Autodesk Inventor part; units mm, degrees
ref_plane "Work Plane1" through (-16.6341, -25.631, 0) normal (0, 0, 1) x (1, 0, 0)
ref_plane "YZ Plane" through (0, 0, 0) normal (1, 0, 0) x (0, 1, 0)
ref_plane "XZ Plane" through (0, 0, 0) normal (0, 1, 0) x (-1, 0, 0)
sketch "Sketch1" plane through (0, 0, 0) normal (0, 1, 0) x (-1, 0, 0)
  line L0 (5.5341, -4.8619) -> (4.7341, -5.0029)
  line L1 (5.5341, -4.4619) -> (5.5341, -4.8619)
  line L2 (4.7341, -4) -> (5.5341, -4.4619)
  line L3 (4.7341, -3.0029) -> (4.7341, -4)
  line L4 (5.5341, -2.8619) -> (4.7341, -3.0029)
  line L5 (5.5341, -2.4619) -> (5.5341, -2.8619)
  line L6 (4.7341, -2) -> (5.5341, -2.4619)
  line L7 (4.7341, -1.0029) -> (4.7341, -2)
  line L8 (5.5341, -0.8619) -> (4.7341, -1.0029)
  line L9 (5.5341, -0.4619) -> (5.5341, -0.8619)
  line L10 (4.7341, 0) -> (5.5341, -0.4619)
  line L11 (10.1341, 0) -> (4.7341, 0)
  line L12 (9.3341, -0.4619) -> (10.1341, 0)
  line L13 (9.3341, -0.8619) -> (9.3341, -0.4619)
  line L14 (10.1341, -1.0029) -> (9.3341, -0.8619)
  line L15 (10.1341, -1.0029) -> (10.1341, -2)
  line L16 (9.3341, -2.4619) -> (10.1341, -2)
  line L17 (9.3341, -2.8619) -> (9.3341, -2.4619)
  line L18 (10.1341, -3.0029) -> (9.3341, -2.8619)
  line L19 (10.1341, -3.0029) -> (10.1341, -4)
  line L20 (9.3341, -4.4619) -> (10.1341, -4)
  line L21 (9.3341, -4.8619) -> (9.3341, -4.4619)
  line L22 (10.1341, -5.0029) -> (9.3341, -4.8619)
  line L23 (10.1341, -5.0029) -> (10.1341, -6)
  line L24 (9.3341, -6.4619) -> (10.1341, -6)
  line L25 (9.3341, -6.8619) -> (9.3341, -6.4619)
  line L26 (10.1341, -7.0029) -> (9.3341, -6.8619)
  line L27 (10.1341, -7.0029) -> (10.1341, -8)
  line L28 (9.3341, -8.4619) -> (10.1341, -8)
  line L29 (9.3341, -8.8619) -> (9.3341, -8.4619)
  line L30 (10.1336, -9.0029) -> (9.3341, -8.8619)
  line L31 (10.1341, -9) -> (10.1341, -10.8672)
  arc A0 (10.1341, -10.8672) -> (10.1663, -11.225) centre (12.1341, -10.8672) ccw
  line L32 (4.5189, -11.225) -> (10.1663, -11.225)
  arc A1 (4.5189, -11.225) -> (4.7341, -10.3226) centre (2.7341, -10.3226) ccw
  line L33 (4.7341, -9) -> (4.7341, -10.3226)
  line L34 (5.5341, -8.8619) -> (4.7346, -9.0029)
  line L35 (5.5341, -8.4619) -> (5.5341, -8.8619)
  line L36 (4.7341, -8) -> (5.5341, -8.4619)
  line L37 (4.7341, -7.0029) -> (4.7341, -8)
  line L38 (5.5341, -6.8619) -> (4.7341, -7.0029)
  line L39 (5.5341, -6.4619) -> (5.5341, -6.8619)
  line L40 (4.7341, -6) -> (5.5341, -6.4619)
  line L41 (4.7341, -5.0029) -> (4.7341, -6)
  line L42 (10.1341, 0) -> (8.6341, 0)
  line L43 (4.7341, 0) -> (6.2341, 0)
  line L44 (6.2341, 0) -> (6.2341, -6)
  line L45 (6.2341, -6) -> (8.6341, -6)
  line L46 (8.6341, -6) -> (8.6341, 0)
  line L47 (8.6341, -6) -> (8.3837, -8.8619)
  line L48 (8.6341, -6) -> (11.5069, -6) construction
  line L49 (6.2341, -6) -> (6.4845, -8.8619)
  line L50 (6.2341, -6) -> (9.1069, -6) construction
  line L51 (6.4845, -8.8619) -> (8.3837, -8.8619)
  line L52 (8.3837, -8.8619) -> (8.2259, -10.666)
  line L53 (8.2259, -10.666) -> (8.1769, -11.225)
  line L54 (6.4845, -8.8619) -> (6.6912, -11.225)
  line L55 (8.6341, 0) -> (6.2341, 0)
  line L56 (6.2341, 0) -> (6.2341, 2)
  line L57 (6.2341, 2) -> (8.6341, 2)
  line L58 (8.6341, 2) -> (8.6341, 0)
  point P0 (0, 0)
  dimension "d0" = 1.5
  dimension "d1" = 1.5
  dimension "d2" = 6
  dimension "d3" = 95
  dimension "d4" = 85
  dimension "d5" = 2
extrude "Extrusion1" add sketch "Sketch1" against normal blind 6.6 contours L56 L57 L58 L11 | L11 L46 L45 L44 | L54 L51 L52 L53 L32 | L45 L47 L51 L49
sketch "Sketch2" plane through (-8.6341, 0, 2) normal (0, 0, 1) x (1, 0, 0)
  circle A0 centre (1.2, 2) radius 0.9
  circle A1 centre (1.2, -8.8) radius 0.9
  circle A2 centre (1.2, 2) radius 2.5
  circle A3 centre (1.2, -8.8) radius 2.5
  line L0 (0, 0) -> (2.4, 0)
  line L1 (0, 0) -> (0, -6.6)
  line L2 (2.4, -6.6) -> (0, -6.6)
  line L3 (2.4, 0) -> (2.4, -6.6)
  line L4 (2.4, 0) -> (2.4, -6.6)
  line L5 (2.4, -6.6) -> (2.4, -6.4)
  line L6 (2.4, -6.4) -> (2.4, -6.087)
  line L7 (0, -6.4) -> (0, -6.0348)
  circle A4 centre (2.9, -6.3282) radius 0.5
  circle A5 centre (-0.5, -6.3282) radius 0.5
  line L8 (0, 0) -> (0, -6.6)
  circle A6 centre (1.2, -8.8) radius 1.1
  circle A7 centre (1.2, 2) radius 1.1
  line L9 (3.9, 0.2) -> (3.9, -6.8)
  line L10 (3.9, -6.8) -> (-1.5, -6.8)
  line L11 (-1.5, -6.8) -> (-1.5, 0.2)
  line L12 (-1.5, 0.2) -> (3.9, 0.2)
  line L13 (-8, -25.631) -> (-8, 3.869)
  line L14 (8.6341, -25.631) -> (-8, -25.631)
  line L15 (8.6341, -25.631) -> (8.6341, 3.869)
  line L16 (-8, 3.869) -> (8.6341, 3.869)
  point P0 (8.6341, 0)
  point P1 (0, -6.3282)
  point P2 (-0.2167, -6.7401)
  point P3 (2.6167, -6.7401)
  point P4 (2.4, -6.3282)
  point P5 (2.4, -0.1932)
  point P6 (0, -0.1932)
  dimension "d16" = 5
  dimension "d17" = 5
  dimension "d19" = 0.2
  dimension "d20" = 1
  dimension "d21" = 1
ref_plane "Work Plane1" through (-16.6341, -25.631, 0) normal (0, 0, 1) x (1, 0, 0)
extrude "Extrusion3" add sketch "Sketch2" along normal blind 1 and the other way blind 2 contours A0 | A1 | A2 L12 L16 | L16 A2 | A2 L3 L0 L1 L12 | L3 L2 A3 L1 A2 | A2 L1 L0 L3 | A4 A3 L2 L3 | L1 L2 A3 A5 | A3 L10 L2 | A3 L10 | L2 A3 | A6 | A7
sketch "Sketch3" plane through (-8.6341, 0, 3) normal (0, 0, 1) x (1, 0, 0)
  circle A0 centre (1.2, -8.8) radius 0.9
  circle A1 centre (1.2, 2) radius 0.9
  point P0 (8.6341, 0)
fillet "Fillet1" radius 0.6 1 edges at (-6.2341, -0.1932, 1.5)
hole "Hole1" at (-7.4341, -8.8, 3) at (-7.4341, 2, 3) direction (0, 0, -1) diameter 2.7 end through all
sketch "Sketch4" plane through (-8.6341, 0, 3) normal (0, 0, 1) x (1, 0, 0)
  arc A0 (2.6516, -0.0354) -> (2.4, -0.5239) centre (3, -0.5239) ccw
  line L0 (3, -0.5239) -> (-1.7059, -0.5239)
  line L1 (-1.7059, -0.5239) -> (-1.7059, 4.8856)
  line L2 (-1.7059, 4.8856) -> (3, 4.8856)
  line L3 (3, 4.8856) -> (3, -0.5239)
  line L4 (3, -0.5239) -> (6.6824, -0.5239)
  line L5 (6.6824, -0.5239) -> (6.6824, 3.9617)
  line L6 (6.6824, 3.9617) -> (3, 3.9617)
  line L7 (3, 3.9617) -> (3, -0.5239)
  point P0 (8.6341, 0)
extrude "Extrusion4" cut sketch "Sketch4" against normal blind 10
properties part number "belt clip 2"
The model under review builds one solid part; all positions refer to its coordinate system, in mm. A direction names the side the tool comes from. Round coordinates to 2 decimals unless told otherwise and drop trailing zeros. Loops run counter-clockwise (first coordinate to the right, second up) from the corner with the lowest first, then second, coordinate; pieces in that order, holes last.
1) Clearance check with flat-ended pins moving along their axes: P1, Ø5, axis at y = -3, z = -8.5, coming from the +X side; P2, Ø3, axis at y = -10, z = -6.5, coming from the +X side; P3, Ø0.7, axis at x = -7.5, z = -5.5, coming from the -Y side; P4, Ø2.5, axis at x = -7.5, y = -10, coming from the -Z side. State where each tip first meets the part, or that it passes through.
Values follow:
P1: stops at x = -6.23
P2: passes through
P3: stops at y = -6.6
P4: stops at z = 0
2) The part is to be moulded in two halves that separate along Y. For faces 4 (the face through (-7, 0, -9)), 5 (the face through (-7.8, -10.1, 1.5)), 6 (the face through (-6.234, -4, -2)), say which applies: pulls with the +Y half, pulls with the -Y half, needs draft (parallel to the pull), parting line crosses it, or undercut.
Values follow:
face 4: pulls with the +Y half
face 5: undercut
face 6: needs draft
3) Tool access review of faces 1 (the face through (-7, -0.524, -2)), 2 (the face through (-7, -6.6, -6)), 3 (the face through (-7, -3, -11.225)): name each direction out of +Z, -Z, +X, -X, +Y, -Y from which nothing blocks a thin tool from reaching the whole face with its end or side.
Values follow:
face 1: +Z, +X, -X, +Y
face 2: -Z, +X, -X, -Y
face 3: -Z, +X, -X, +Y, -Y
4) Consider section A-A on y = -8.8. State the section outline as (x, z) points.
Values follow:
outline: (-9.93, 0) - (-8.78, 0) - (-8.78, 3) - (-9.93, 3) - close; (-6.08, 0) - (-4.93, 0) - (-4.93, 3) - (-6.08, 3) - close
5) Consider section B-B on z = 1.25. State the section outline as (x, y) points.
Values follow:
outline: (-8.85, -6.74) arc R2.5 ccw (long way) to (-6.02, -6.74) arc R0.5 cw to (-6.23, -6.33) - (-6.23, -0.52) - (-8.63, -0.52) - (-8.63, -6.33) arc R0.5 cw to start; hole circle Ø2.7 at (-7.43, -8.8)
6) Consider section C-C on y = -3.5. State the section outline as (x, z) points (1 decimal), then the cut area to 3 significant figures.
Values follow:
outline: (-8.6, -6) - (-8.4, -8.9) - (-8.2, -10.7) - (-8.2, -11.2) - (-6.7, -11.2) - (-6.5, -8.9) - (-6.2, -6) - (-6.2, 3) - (-8.6, 3) - close
area: 31.8 mm2
7) Wall thickness on line 1 along X through (y, z) = (-8.8, 0.7); line 2 along Y through (x, z) = (-8.15, -2); line 3 along Y through (x, z) = (-6.65, 1.5): over which ranges is each line inside the solid? List them lowest first.
Values follow:
line 1: x = -9.93 to -8.78, -6.08 to -4.93
line 2: y = -6.6 to -0.52
line 3: y = -11.17 to -9.9, -7.7 to -0.52
8) Consider section D-D on x = -6.85. State the section outline as (y, z) points (3 decimals).
Values follow:
outline: (-11.231, 0) - (-10.017, 0) - (-10.017, 3) - (-11.231, 3) - close; (-7.583, 0) - (-6.6, 0) - (-6.6, -11.225) - (0, -11.225) - (0, -7) - (-0.524, -7) - (-0.524, 3) - (-7.583, 3) - close
